Here's how the part is built. I have some questions about the finished solid (model axes, mm). Coordinates: 2 decimals unless noted, no trailing zeros. Write each loop counter-clockwise with the first axis right and the second up, starting at its lowest first coordinate (ties: lowest second). Pieces come first, ordered by that corner, then holes.
```python
from build123d import *

# Parameters (mm, degrees)
BOSS_EXTRUDE1_DEPTH = 10
SKETCH3_R           = 5
SKETCH3_R_2         = 2.1
CUT_EXTRUDE1_DEPTH  = 10


with BuildPart() as part:
    # Sketch2 → Boss-Extrude1 (new body)
    with BuildSketch(Plane(origin=(0, 0, 0), x_dir=(1, 0, 0), z_dir=(0, 1, 0))):
        with BuildLine():
            Line((-224.228087349, 94.161183877), (85.275800554, 94.161183877))
            ThreePointArc((85.275800554, 94.161183877), (115.275800554, 64.161183877), (85.275800554, 34.161183877))
            Line((85.275800554, 34.161183877), (-189.724199446, 34.161183877))
            Line((-189.724199446, 34.161183877), (-216.678540206, 34.162870649))
            ThreePointArc((-216.678540206, 34.162870649), (-250.480097378, 40.753794505), (-279.331674578, 59.557305814))
            Line((-279.331674578, 59.557305814), (-303.368494474, 83.28636858))
            ThreePointArc((-303.368494474, 83.28636858), (-300.074671731, 139.135756578), (-247.333786879, 120.470214177))
            Line((-247.333786879, 120.470214177), (-236.884563066, 101.993319193))
            ThreePointArc((-236.884563066, 101.993319193), (-227.511529016, 96.189234726), (-216.67478541, 94.162870531))
            Line((-216.67478541, 94.162870531), (-224.228087349, 94.161183877))
        make_face()
    extrude(amount=BOSS_EXTRUDE1_DEPTH)

    # Sketch3 → Cut-Extrude1 (cut)
    with BuildSketch(Plane(origin=(0, 10, 0), x_dir=(1, 0, 0), z_dir=(0, 1, 0))):
        with Locations(Location((-280.722408111, 109.972596722, 0), (0, 0, 270))):
            Circle(SKETCH3_R)
        with Locations(Location((-280.722408111, 139.972596722, 0), (0, 0, 270))):
            Circle(SKETCH3_R_2)
        with Locations(Location((-310.722408111, 109.972596722, 0), (0, 0, 270))):
            Circle(SKETCH3_R_2)
        with Locations(Location((-280.722408111, 79.972596722, 0), (0, 0, 270))):
            Circle(SKETCH3_R_2)
        with Locations(Location((-250.722408111, 109.972596722, 0), (0, 0, 270))):
            Circle(SKETCH3_R_2)
    extrude(amount=-CUT_EXTRUDE1_DEPTH, mode=Mode.SUBTRACT)


solid = part.part
```
1) Imagine slicing it at A-A on y = 4.75. Please give me the cut outline in (x, z).
Values follow:
outline: (-303.37, -83.29) arc R35 ccw (long way) to (-247.33, -120.47) - (-236.88, -101.99) arc R30 cw to (-216.67, -94.16) - (-224.23, -94.16) - (85.28, -94.16) arc R30 ccw to (85.28, -34.16) - (-189.72, -34.16) - (-216.68, -34.16) arc R90 ccw to (-279.33, -59.56) - close; hole circle Ø4.2 at (-310.72, -109.97); hole circle Ø10 at (-280.72, -109.97); hole circle Ø4.2 at (-280.72, -139.97); hole circle Ø4.2 at (-280.72, -79.97); hole circle Ø4.2 at (-250.72, -109.97)
2) Imagine slicing it at B-B on x = 3. Please give me the cut outline in (y, z).
Values follow:
outline: (0, -94.16) - (10, -94.16) - (10, -34.16) - (0, -34.16) - close
3) Will these pins go through, and if not, where does the flat tip stop? pin 1 (5.5 mm diameter, centred on x = -280.72, z = -139.97, fed in from +Y); pin 2 (5 mm diameter, centred on x = 23, y = 3.5, fed in from -Z); pin 3 (1 mm diameter, centred on y = 4, z = -70, fed in from -X); pin 4 (6 mm diameter, centred on y = 7, z = -64.5, fed in from -X).
Values follow:
pin 1: stops at y = 10
pin 2: stops at z = -94.16
pin 3: stops at x = -290.42
pin 4: stops at x = -287.38
4) We'd pull the mould along Z, two halves only. Please class faces 1 (the face through (-283.765, 5.07, -113.94)), 2 (the face through (-97, 0, -78)), 3 (the face through (-227.656, 4.93, -96.246)): pulls with the +Z half, pulls with the -Z half, needs draft (parallel to the pull), parting line crosses it, or undercut.
Values follow:
face 1: undercut
face 2: needs draft
face 3: pulls with the -Z half
5) I need wall thicknesses on probe 1 along Z at (x, y) = (-279, 8.25); probe 2 along Z at (x, y) = (-151, 8); probe 3 along X at (y, z) = (3.25, -107.5). Which ranges of each line are inside material? Lowest first, please.
Values follow:
probe 1: z = -144.93 to -141.17, -138.77 to -114.67, -105.28 to -81.17, -78.77 to -59.24
probe 2: z = -94.16 to -34.16
probe 3: x = -315.63 to -285.07, -276.38 to -240
6) Imagine slicing it at C-C on z = -50.5. Please give me the cut outline in (x, y).
Values follow:
outline: (-268.38, 0) - (111.98, 0) - (111.98, 10) - (-268.38, 10) - close
